```python
from build123d import *

# Parameters (mm, degrees)
SKETCH1_W                 = 69.296350976
SKETCH1_H                 = 69.296350976
SKETCH1_W_2               = 49.515978472
SKETCH1_H_2               = 50
BOSS_EXTRUDE1_DEPTH       = 2
SKETCH2_R                 = 30
BOSS_EXTRUDE2_DEPTH       = 70
BOSS_EXTRUDE2_TAPER       = -5
SKETCH3_R                 = 36.124206447
BOSS_EXTRUDE3_DEPTH       = 20
SKETCH4_R                 = 28
CUT_EXTRUDE2_DEPTH        = 20
SKETCH5_W                 = 30
SKETCH5_H                 = 50
BOSS_EXTRUDE4_DEPTH       = 50
SKETCH6_W                 = 50
SKETCH6_H                 = 30
BOSS_EXTRUDE5_DEPTH       = 40
FILLET1_R                 = 20
BOSS_EXTRUDE11_DEPTH      = 70
CUT_EXTRUDE22_DEPTH       = 70
CUT_EXTRUDE22_DEPTH_BACK  = 70
SKETCH22_R                = 5
BOSS_EXTRUDE12_DEPTH      = 51
BOSS_EXTRUDE12_DEPTH_BACK = 2


with BuildPart() as part:
    # Sketch1 → Boss-Extrude1 (new body)
    with BuildSketch(Plane(origin=(0, 0, 0), x_dir=(1, 0, 0), z_dir=(0, 1, 0))):
        Rectangle(SKETCH1_W, SKETCH1_H)
        with Locations((59.406164724, 0)):
            Rectangle(SKETCH1_W_2, SKETCH1_H_2)
    extrude(amount=BOSS_EXTRUDE1_DEPTH)

    # Sketch2 → Boss-Extrude2 (add)
    with BuildSketch(Plane(origin=(0, 2, 0), x_dir=(1, 0, 0), z_dir=(0, 1, 0))):
        Circle(SKETCH2_R)
    extrude(amount=BOSS_EXTRUDE2_DEPTH, taper=BOSS_EXTRUDE2_TAPER)

    # Sketch3 → Boss-Extrude3 (add)
    with BuildSketch(Plane(origin=(0, 72, 0), x_dir=(1, 0, 0), z_dir=(0, 1, 0))):
        Circle(SKETCH3_R)
    extrude(amount=BOSS_EXTRUDE3_DEPTH)

    # Sketch4 → Cut-Extrude2 (cut)
    with BuildSketch(Plane(origin=(0, 92, 0), x_dir=(1, 0, 0), z_dir=(0, 1, 0))):
        Circle(SKETCH4_R)
    extrude(amount=-CUT_EXTRUDE2_DEPTH, mode=Mode.SUBTRACT)

    # Sketch5 → Boss-Extrude4 (add)
    with BuildSketch(Plane(origin=(0, 2, 0), x_dir=(1, 0, 0), z_dir=(0, 1, 0))):
        with Locations((69.16415396, 0)):
            Rectangle(SKETCH5_W, SKETCH5_H)
    extrude(amount=BOSS_EXTRUDE4_DEPTH)

    # Sketch6 → Boss-Extrude5 (add)
    with BuildSketch(Plane.ZY.offset(-54.16415396)):
        with Locations((0, 37)):
            Rectangle(SKETCH6_W, SKETCH6_H)
    extrude(amount=BOSS_EXTRUDE5_DEPTH)

    # Fillet1
    fillet1_edges = [part.edges().sort_by_distance(p)[0] for p in [
        (84.16415396, 52, 0),
    ]]
    fillet(fillet1_edges, radius=FILLET1_R)

    # Sketch7 → Boss-Extrude11 (add)
    with BuildSketch(Plane(origin=(0, 92, 0), x_dir=(1, 0, 0), z_dir=(0, 1, 0))):
        with BuildLine():
            Line((27.734618886, 23.14625686), (38.570246087, 23.14625686))
            Line((38.570246087, 23.14625686), (38.570246087, 33.14625686))
            Line((38.570246087, 33.14625686), (14.36258847, 33.14625686))
            ThreePointArc((14.36258847, 33.14625686), (21.634318034, 28.929475879), (27.734618886, 23.14625686))
        make_face()
        with BuildLine():
            ThreePointArc((-14.36258847, 33.14625686), (-21.634318034, 28.929475879), (-27.734618886, 23.14625686))
            Line((-27.734618886, 23.14625686), (-15.755976433, 23.14625686))
            ThreePointArc((-15.755976433, 23.14625686), (0, 28), (15.755976433, 23.14625686))
            Line((15.755976433, 23.14625686), (27.734618886, 23.14625686))
            ThreePointArc((27.734618886, 23.14625686), (21.634318034, 28.929475879), (14.36258847, 33.14625686))
            Line((14.36258847, 33.14625686), (-14.36258847, 33.14625686))
        make_face()
        with BuildLine():
            Line((-37.772768209, 23.14625686), (-27.734618886, 23.14625686))
            ThreePointArc((-27.734618886, 23.14625686), (-21.634318034, 28.929475879), (-14.36258847, 33.14625686))
            Line((-14.36258847, 33.14625686), (-37.772768209, 33.14625686))
            Line((-37.772768209, 33.14625686), (-37.772768209, 23.14625686))
        make_face()
        with BuildLine():
            ThreePointArc((14.36258847, 33.14625686), (0, 36.124206447), (-14.36258847, 33.14625686))
            Line((-14.36258847, 33.14625686), (14.36258847, 33.14625686))
        make_face()
        with BuildLine():
            ThreePointArc((15.755976433, 23.14625686), (0, 28), (-15.755976433, 23.14625686))
            Line((-15.755976433, 23.14625686), (15.755976433, 23.14625686))
        make_face()
        with BuildLine():
            Line((-37.772768209, -33.14625686), (-14.36258847, -33.14625686))
            ThreePointArc((-14.36258847, -33.14625686), (-21.634318034, -28.929475879), (-27.734618886, -23.14625686))
            Line((-27.734618886, -23.14625686), (-37.772768209, -23.14625686))
            Line((-37.772768209, -23.14625686), (-37.772768209, -33.14625686))
        make_face()
        with BuildLine():
            Line((-14.36258847, -33.14625686), (14.36258847, -33.14625686))
            ThreePointArc((14.36258847, -33.14625686), (21.634318034, -28.929475879), (27.734618886, -23.14625686))
            Line((27.734618886, -23.14625686), (15.755976433, -23.14625686))
            ThreePointArc((15.755976433, -23.14625686), (0, -28), (-15.755976433, -23.14625686))
            Line((-15.755976433, -23.14625686), (-27.734618886, -23.14625686))
            ThreePointArc((-27.734618886, -23.14625686), (-21.634318034, -28.929475879), (-14.36258847, -33.14625686))
        make_face()
        with BuildLine():
            ThreePointArc((27.734618886, -23.14625686), (21.634318034, -28.929475879), (14.36258847, -33.14625686))
            Line((14.36258847, -33.14625686), (38.570246087, -33.14625686))
            Line((38.570246087, -33.14625686), (38.570246087, -23.14625686))
            Line((38.570246087, -23.14625686), (27.734618886, -23.14625686))
        make_face()
        with BuildLine():
            ThreePointArc((-15.755976433, -23.14625686), (0, -28), (15.755976433, -23.14625686))
            Line((15.755976433, -23.14625686), (-15.755976433, -23.14625686))
        make_face()
        with BuildLine():
            ThreePointArc((-14.36258847, -33.14625686), (0, -36.124206447), (14.36258847, -33.14625686))
            Line((14.36258847, -33.14625686), (-14.36258847, -33.14625686))
        make_face()
    extrude(amount=BOSS_EXTRUDE11_DEPTH)

    # Sketch20 → Cut-Extrude22 (cut, two sides)
    with BuildSketch(Plane.XY.offset(33.14625686)) as cut_extrude22_sk:
        with BuildLine():
            Line((-14.36258847, 92), (-14.36258847, 112.655146554))
            ThreePointArc((-14.36258847, 112.655146554), (-1.971914178, 158.039808748), (17.401848907, 115.168446794))
            ThreePointArc((17.401848907, 115.168446794), (15.153696147, 111.886989388), (14.36258847, 107.988745913))
            Line((14.36258847, 107.988745913), (14.36258847, 92))
            Line((14.36258847, 92), (38.570246087, 92))
            Line((38.570246087, 92), (38.570246087, 162))
            Line((38.570246087, 162), (-37.772768209, 162))
            Line((-37.772768209, 162), (-37.772768209, 92))
            Line((-37.772768209, 92), (-14.36258847, 92))
        make_face()
    extrude(amount=CUT_EXTRUDE22_DEPTH, mode=Mode.SUBTRACT)
    extrude(cut_extrude22_sk.sketch, amount=-CUT_EXTRUDE22_DEPTH_BACK, mode=Mode.SUBTRACT)

    # Sketch22 → Boss-Extrude12 (add, two sides)
    with BuildSketch(Plane.XY.offset(-23.14625686)) as boss_extrude12_sk:
        with Locations((0, 133.117698996)):
            Circle(SKETCH22_R)
    extrude(amount=BOSS_EXTRUDE12_DEPTH)
    extrude(boss_extrude12_sk.sketch, amount=-BOSS_EXTRUDE12_DEPTH_BACK)


solid = part.part
```
Design review of the part built by this model. Coordinates are the model's own, in mm. A direction names the side the tool comes from. Give positions to 0.01 mm unless a question says otherwise; leave off trailing zeros. Order: outer loops, then holes, each group sorted by start corner. A loop starts at its lowest first (then second) coordinate and runs counter-clockwise, first axis right, second up. Notation, with made-up numbers: (65, 35) - (71, 35) arc R11 ccw to (71, 44) - close; hole circle Ø3 at (21, 1.25). An arc over 180 degrees is marked (long way). Use a Markdown table: item, result. Add a question column.
(1) Wall thickness on probe 1 along Y at (x, z) = (53, -9); probe 2 along Z at (x, y) = (0, 79); probe 3 along Y at (x, z) = (62, 16.5): over which ranges is each line inside the solid? List them lowest first. Write a range as [from, to].
(2) Mouldability with a two-part tool opening along Y and no side actions: class faces 5 (the face through (78.461, 45.986, -0.35)), 6 (the face through (19, 136, -33.146)), 7 (the face through (14.363, 100, -28)) as +Y half, -Y half, draft (parallel to the pull), parting line (faces both ways), or undercut.
(3) Add section C-C on z = -12.5. Give the number of separate pieces and of enclosed holes in the cut face, then the cut area to 3 significant figures.
(4) Machinability: for faces 1 (the face through (54.164, 12, 0)), 2 (the face through (0, 92, 25)), 3 (the face through (18, 136, 33.146)), 4 (the face through (-18, 133, -33.146)), which of the approach directions +Z, -Z, +X, -X, +Y, -Y give a long, thin tool a straight path to every point of the face, cutting with its end or side? Answer none if there is none.
(5) Add section A-A on y = 100.5. Give the boundary of the cut face in (x, z).
(6) Clearance check with flat-ended pins moving along their axes: P1, Ø3, axis at x = -18.5, y = 132, coming from the -Z side; P2, Ø0.6, axis at x = 11.5, y = 0.5, coming from the +Z side; P3, Ø3, axis at y = 101, z = -29.5, coming from the -X side. State where each tip first meets the part, or that it passes through.
(7) Add section B-B on x = 0. Give the boundary of the cut face in (y, z), then the cut area to 3 significant figures.
(8) Add section D-D on y = 141. Give the boundary of the cut face in (x, z).
Report:
| question | item | result |
|---|---|---|
| 1 | probe 1 | y = [0, 2], [22, 52] |
| 1 | probe 2 | z = [-36.12, -28], [28, 36.12] |
| 1 | probe 3 | y = [0, 52] |
| 2 | face 5 | +Y half |
| 2 | face 6 | draft |
| 2 | face 7 | undercut |
| 3 | separate pieces | 2 |
| 3 | enclosed holes | 1 |
| 3 | area | 7,070 mm² |
| 4 | face 1 | +Z, -Z |
| 4 | face 2 | none |
| 4 | face 3 | +Z, +X, +Y |
| 4 | face 4 | -Z, -X, +Y |
| 5 | outline | (-14.36, -33.15) arc R36.12 ccw to (14.36, -33.15) - (14.36, -23.15) - (-14.36, -23.15) - close; (-14.36, 23.15) - (14.36, 23.15) - (14.36, 33.15) arc R36.12 ccw to (-14.36, 33.15) - close |
| 6 | P1 | stops at z = -33.15 |
| 6 | P2 | stops at z = 34.65 |
| 6 | P3 | stops at x = -14.36 |
| 7 | outline | (0, -34.65) - (2, -34.65) - (2, -30) - (72, -36.12) - (158.12, -36.12) - (158.12, -23.15) - (138.12, -23.15) - (138.12, 23.15) - (158.12, 23.15) - (158.12, 36.12) - (72, 36.12) - (2, 30) - (2, 34.65) - (0, 34.65) - close; hole (72, -28) - (92, -28) - (92, -23.15) - (128.12, -23.15) - (128.12, 23.15) - (92, 23.15) - (92, 28) - (72, 28) - close |
| 7 | area | 7,270 mm² |
| 8 | outline | (-23.72, -33.15) - (-14.36, -33.15) arc R36.12 ccw to (14.36, -33.15) - (23.72, -33.15) - (23.72, -23.15) - (-23.72, -23.15) - close; (-23.72, 23.15) - (23.72, 23.15) - (23.72, 33.15) - (14.36, 33.15) arc R36.12 ccw to (-14.36, 33.15) - (-23.72, 33.15) - close |
